Can you work these out from the model? Positions are in its coordinate system, mm. A direction names the side the tool comes from. Coordinates: 2 decimals unless noted, no trailing zeros. Write each loop counter-clockwise with the first axis right and the second up, starting at its lowest first coordinate (ties: lowest second). Pieces come first, ordered by that corner, then holes. Notation, with made-up numbers: (17.5, 22.5) -> (33.5, 22.5) arc R16 cw to (33.5, 48.5) -> close; hole circle Ø10 at (-32, 48.25). An arc over 180 degrees is marked (long way). Use one line per item in the form item = value.
```python
from build123d import *

# Parameters (mm, degrees)
BOSS_EXTRUDE1_DEPTH            = 9
SKETCH4_W                      = 18
SKETCH4_H                      = 44.313566923
CUT_EXTRUDE3_DEPTH             = 6
FILLET1_R                      = 0.5
CUT_EXTRUDE4_DEPTH             = 20
CUT_EXTRUDE5_DEPTH             = 19.0000001
BOSS_EXTRUDE2_DEPTH            = 18
FILLET2_R                      = 3
SKETCH11_OUTSIDE_W             = 65.077
SKETCH11_OUTSIDE_H             = 50.285
SKETCH11_OUTSIDE_W_2           = 10
SKETCH11_OUTSIDE_H_2           = 20
CUT_EXTRUDE6_DEPTH             = 19.0000001
F_2_56_TAPPED_HOLE1_D          = 1.778
F_2_56_TAPPED_HOLE1_DEPTH      = 5.73
F_2_56_TAPPED_HOLE1_TIP        = 0.53416509
CUT_EXTRUDE7_DEPTH             = 2.2
F_1_16_0_0625_DIAMETER_HOLE1_D = 1.5875


with BuildPart() as part:
    # Sketch1 → Boss-Extrude1 (new body, symmetric)
    with BuildSketch(Plane(origin=(0, 0, 0), x_dir=(0, 0, -1), z_dir=(1, 0, 0))):
        with BuildLine():
            Line((3.00520382, -3.00520382), (20, 13.98959236))
            Line((20, 13.98959236), (20, 30))
            Line((20, 30), (0, 30))
            Line((0, 30), (0, -4.25))
            ThreePointArc((0, -4.25), (1.626404588, -3.926488013), (3.00520382, -3.00520382))
        make_face()
    extrude(amount=BOSS_EXTRUDE1_DEPTH, both=True)

    # Sweep1: sweep along a path in Sketch2
    with BuildLine(Plane(origin=(0, 0, 0), x_dir=(0, 0, -1), z_dir=(1, 0, 0))) as sweep1_path:
        Line((20, 13.98959236), (3.00520382, -3.00520382))
        ThreePointArc((3.00520382, -3.00520382), (1.626404588, -3.926488013), (0, -4.25))
    # Sketch3 → Sweep1 (sweep)
    with BuildSketch(Plane.XY):
        with BuildLine():
            Line((9, -4.25), (-9, -4.25))
            Line((-9, -4.25), (-9, -6.701215317))
            ThreePointArc((-9, -6.701215317), (0, -4.65), (9, -6.701215317))
            Line((9, -6.701215317), (9, -4.25))
        make_face()
    sweep(path=sweep1_path.line)

    # Sketch4 → Cut-Extrude3 (cut)
    with BuildSketch(Plane(origin=(0, 0, -20), x_dir=(-1, 0, 0), z_dir=(0, 0, -1))):
        with Locations((0, 7.843216539)):
            Rectangle(SKETCH4_W, SKETCH4_H)
    extrude(amount=CUT_EXTRUDE3_DEPTH, mode=Mode.SUBTRACT)

    # Fillet1
    fillet1_edges = [part.edges().sort_by_distance(p)[0] for p in [
        (9, 2.89228781, -12.369237397),
        (-9, 2.89228781, -12.369237397),
        (9, -6.191115675, -2.564444079),
        (-9, -6.191115675, -2.564444079),
    ]]
    fillet(fillet1_edges, radius=FILLET1_R)

    # Mirror1: part across plane


with BuildPart() as part_1:
    add(part.part)
    add(part.part.mirror(Plane(origin=(9, 30, 0), x_dir=(1, 0, 0), z_dir=(0, 0, -1))))

    # Sketch5 → Cut-Extrude4 (cut, symmetric)
    with BuildSketch(Plane(origin=(0, 0, 0), x_dir=(0, 0, -1), z_dir=(1, 0, 0))):
        Polygon((20, 16), (-7.485561137, 10.657348129), (-11.245391787, 30), (20, 30), align=None)
    extrude(amount=CUT_EXTRUDE4_DEPTH, both=True, mode=Mode.SUBTRACT)

    # Sketch8 → Cut-Extrude5 (cut, through all)
    with BuildSketch(Plane.ZY.offset(9)):
        Polygon((10.6659344, 27.018950173), (20, 28), (20, 30), (11.245391787, 30), align=None)
    extrude(amount=-CUT_EXTRUDE5_DEPTH, mode=Mode.SUBTRACT)

    # Sketch10 → Boss-Extrude2 (add)
    with BuildSketch(Plane.ZY.offset(9)):
        Polygon((20, 28), (29.945218954, 29.045284633), (30.258804343, 26.061718947), (20, 24.983475161), align=None)
    extrude(amount=-BOSS_EXTRUDE2_DEPTH)

    # Fillet2
    fillet2_edges = [part_1.edges().sort_by_distance(p)[0] for p in [
        (0, 24.983475161, 20),
        (0, 10.657348129, 7.485561137),
    ]]
    fillet(fillet2_edges, radius=FILLET2_R)

    # Sketch11 outside → Cut-Extrude6 (cut, through all)
    with BuildSketch(Plane.ZY.offset(9)):
        with Locations((5.1295, 11.3115)):
            Rectangle(SKETCH11_OUTSIDE_W, SKETCH11_OUTSIDE_H)
        with Locations((0, -8)):
            Rectangle(SKETCH11_OUTSIDE_W_2, SKETCH11_OUTSIDE_H_2, mode=Mode.SUBTRACT)
    extrude(amount=-CUT_EXTRUDE6_DEPTH, mode=Mode.SUBTRACT)

    # Sketch13 → Revolve1 (revolve)
    with BuildSketch(Plane(origin=(0, 0, 0), x_dir=(0, 0, -1), z_dir=(1, 0, 0))):
        Polygon((0, 2), (0, 5.9), (-4.9, 5.9), (-4.9, 3.9), (-3, 3.9), (-3, 2), align=None)
    revolve(axis=Axis((0, 0, 0), (0, -1, 0)))

    # #2-56 Tapped Hole1
    with Locations(Plane(origin=(0, 5.9, 0), x_dir=(1, 0, 0), z_dir=(0, 1, 0))):
        with Locations((0, 0)):
            Hole(F_2_56_TAPPED_HOLE1_D / 2, depth=F_2_56_TAPPED_HOLE1_DEPTH)
            with Locations((0, 0, -(F_2_56_TAPPED_HOLE1_DEPTH + F_2_56_TAPPED_HOLE1_TIP / 2))):  # 118° drill point
                Cone(0, F_2_56_TAPPED_HOLE1_D / 2, F_2_56_TAPPED_HOLE1_TIP, mode=Mode.SUBTRACT)

    # Sketch16 → Cut-Extrude7 (cut)
    with BuildSketch(Plane.XY.offset(5)):
        with BuildLine():
            Line((1.7, 7.96125108), (1.7, 1))
            ThreePointArc((1.7, 1), (0, -0.7), (-1.7, 1))
            Line((-1.7, 1), (-1.7, 7.96125108))
            ThreePointArc((-1.7, 7.96125108), (0, 9.66125108), (1.7, 7.96125108))
        make_face()
    extrude(amount=-CUT_EXTRUDE7_DEPTH, mode=Mode.SUBTRACT)

    # 1/16 (0.0625) Diameter Hole1 (through all)
    with Locations(Plane.XY.offset(2.8)):
        with Locations((0, 0.853308914)):
            Hole(F_1_16_0_0625_DIAMETER_HOLE1_D / 2)


solid = part_1.part
```
Q1. If I drill on line 1 (Z direction, x = 0, y = 2.25); line 2 (X direction, y = 0, z = 4.5); line 3 (Y direction, x = -3.75, z = -2.5), over which ranges is the centre line in solid material (lowest first)? Write a range as from..to.
Return value:
line_1 = -3..-0.89, 0.89..2.8
line_2 = -9..-1.37, 1.37..9
line_3 = -4.32..2, 3.9..5.9
Q2. Will these pins go through, and if not, where does the flat tip stop? pin 1 (3 mm diameter, centred on x = 0, z = 0, fed in from -Y); pin 2 (1.4 mm diameter, centred on y = 5, z = 3.5, fed in from -X); pin 3 (3 mm diameter, centred on x = 0.5, z = -2, fed in from -Y).
Return value:
pin_1 = -4.7
pin_2 = -4.02
pin_3 = -4.64
Q3. Thinking about a two-plate mould opening in X: for faces 1 (the flat face through (-0.1, 3.9, -3.4)), 2 (the cylindrical face through (-0.82, 3.63, 0.34)), 3 (the flat face through (9, -2, 0)), 4 (the flat face through (1.7, 1.5, 3.9)), which applies, released by +X, released by -X, zero draft, split by the parting line, or undercut?
Return value:
face_1 = zero draft
face_2 = undercut
face_3 = released by +X
face_4 = undercut
Q4. For faces 5 (the cylindrical face through (-0.191, 4.886, -4.896)), 6 (the flat face through (-1.7, 5, 4)), 7 (the cylindrical face through (0, 3, -3)), which set-ups out of +Z, -Z, +X, -X, +Y, -Y let a thin tool reach every point of the face, with its end or its side?
Return value:
face_5 = +Y
face_6 = +Z, +Y
face_7 = none
Q5. Suppose I cut it at A-A (y = 0.5). Write out the boundary of the cut face in (x, z), then the cut area to 3 significant figures.
Return value:
outline = (-9, -5) -> (-0.71, -5) -> (-0.71, -0.53) arc R0.89 cw to (-0.71, 0.53) -> (-0.71, 2.8) -> (-1.62, 2.8) -> (-1.62, 5) -> (-9, 5) -> close; (0.71, -5) -> (9, -5) -> (9, 5) -> (1.62, 5) -> (1.62, 2.8) -> (0.71, 2.8) -> (0.71, 0.53) arc R0.89 cw to (0.71, -0.53) -> close
area = 162 mm2
